from build123d import *

# Parameters (mm, degrees)
SKETCH1_R           = 17.5
BOSS_EXTRUDE1_DEPTH = 3
SKETCH2_R           = 2.735
SKETCH2_R_2         = 0.5
CUT_EXTRUDE1_DEPTH  = 3
SKETCH3_R           = 1.5
CUT_EXTRUDE2_DEPTH  = 3


with BuildPart() as part:
    # Sketch1 → Boss-Extrude1 (new body)
    with BuildSketch(Plane.XY):
        Circle(SKETCH1_R)
    extrude(amount=BOSS_EXTRUDE1_DEPTH)

    # Sketch2 → Cut-Extrude1 (cut)
    with BuildSketch(Plane.XY.offset(3)):
        with Locations((0, -5.5)):
            Circle(SKETCH2_R)
        with Locations((0, 14.5)):
            Circle(SKETCH2_R_2)
        with Locations((-9, 3.8)):
            Circle(SKETCH2_R)
        with Locations((9, 3.8)):
            Circle(SKETCH2_R)
    extrude(amount=-CUT_EXTRUDE1_DEPTH, mode=Mode.SUBTRACT)

    # Sketch3 → Cut-Extrude2 (cut)
    with BuildSketch(Plane.XY.offset(3)):
        with Locations((0, 7.5)):
            Circle(SKETCH3_R)
        with Locations((0, 2.5)):
            Circle(SKETCH3_R)
    extrude(amount=-CUT_EXTRUDE2_DEPTH, mode=Mode.SUBTRACT)


solid = part.part
The listing builds one solid part. Answer for the finished solid, in the listing's coordinates (mm). Coordinates: 2 decimals unless noted, no trailing zeros. Loops run counter-clockwise (first coordinate to the right, second up) from the corner with the lowest first, then second, coordinate; pieces in that order, holes last. Notation, with made-up numbers: M 36,3.25 L 91,3.25 A15 ccw 91,23.25 Z; hole C 42,75.5 d1. An arc over 180 degrees is marked long. Answer in a Markdown table with one row per item.
1) Find section D-D (y = 2.5). Determine the outline of the cut face in (x, z), then the cut area to 3 significant figures.
Answers below:
| item | result |
|---|---|
| outline | M -17.32,0 L -11.41,0 L -11.41,3 L -17.32,3 Z; M -6.59,0 L -1.5,0 L -1.5,3 L -6.59,3 Z; M 1.5,0 L 6.59,0 L 6.59,3 L 1.5,3 Z; M 11.41,0 L 17.32,0 L 17.32,3 L 11.41,3 Z |
| area | 66.0 mm^2 |
2) Find section B-B (x = 1). Determine the outline of the cut face in (y, z).
Answers below:
| item | result |
|---|---|
| outline | M -17.47,0 L -8.05,0 L -8.05,3 L -17.47,3 Z; M -2.95,0 L 1.38,0 L 1.38,3 L -2.95,3 Z; M 3.62,0 L 6.38,0 L 6.38,3 L 3.62,3 Z; M 8.62,0 L 17.47,0 L 17.47,3 L 8.62,3 Z |
3) Find the intervals of material crossed by probe 1 along Y at (x, z) = (0, 2) (3 decimals); probe 2 along X at (y, z) = (4.5, 1.95); probe 3 along X at (y, z) = (2, 1.7), in increasing order.
Answers below:
| item | result |
|---|---|
| probe 1 | -17.5 to -8.235, -2.765 to 1, 4 to 6, 9 to 14, 15 to 17.5 |
| probe 2 | -16.91 to -11.64, -6.36 to 6.36, 11.64 to 16.91 |
| probe 3 | -17.39 to -11.06, -6.94 to -1.41, 1.41 to 6.94, 11.06 to 17.39 |
4) Determine the mould class of faces 1 (the cylindrical face through (-6.39, 4.62, 1.52)), 2 (the flat face through (0, 0, 0)), 3 (the cylindrical face through (-13.887, -10.648, 1.479)), 4 (the cylindrical face through (0, 15, 2)) for opening direction X: released by +X, released by -X, zero draft, split by the parting line, or undercut.
Answers below:
| item | result |
|---|---|
| face 1 | undercut |
| face 2 | zero draft |
| face 3 | split by the parting line |
| face 4 | undercut |
5) Find section A-A (z = 2.4). Determine the outline of the cut face in (x, y) (3 decimals).
Answers below:
| item | result |
|---|---|
| outline | C 0,0 d35; hole C -9,3.8 d5.47; hole C 0,-5.5 d5.47; hole C 0,2.5 d3; hole C 0,7.5 d3; hole C 0,14.5 d1; hole C 9,3.8 d5.47 |
6) Find section C-C (y = 7.5). Determine the outline of the cut face in (x, z), then the cut area to 3 significant figures.
Answers below:
| item | result |
|---|---|
| outline | M -15.81,0 L -1.5,0 L -1.5,3 L -15.81,3 Z; M 1.5,0 L 15.81,0 L 15.81,3 L 1.5,3 Z |
| area | 85.9 mm^2 |
